Drawing for the job (mm, zero at the part's lowest x, y, z). Coordinates: 2 decimals unless noted, no trailing zeros. Write each loop counter-clockwise with the first axis right and the second up, starting at its lowest first coordinate (ties: lowest second). Pieces come first, ordered by that corner, then holes. Notation, with made-up numbers: (50, 33) - (67, 33) arc R26 cw to (67, 49) - close; hole circle Ø3 at (-34.5, -31.75). An arc over 180 degrees is marked (long way). Write each question's results on one line, items separated by ' | '.
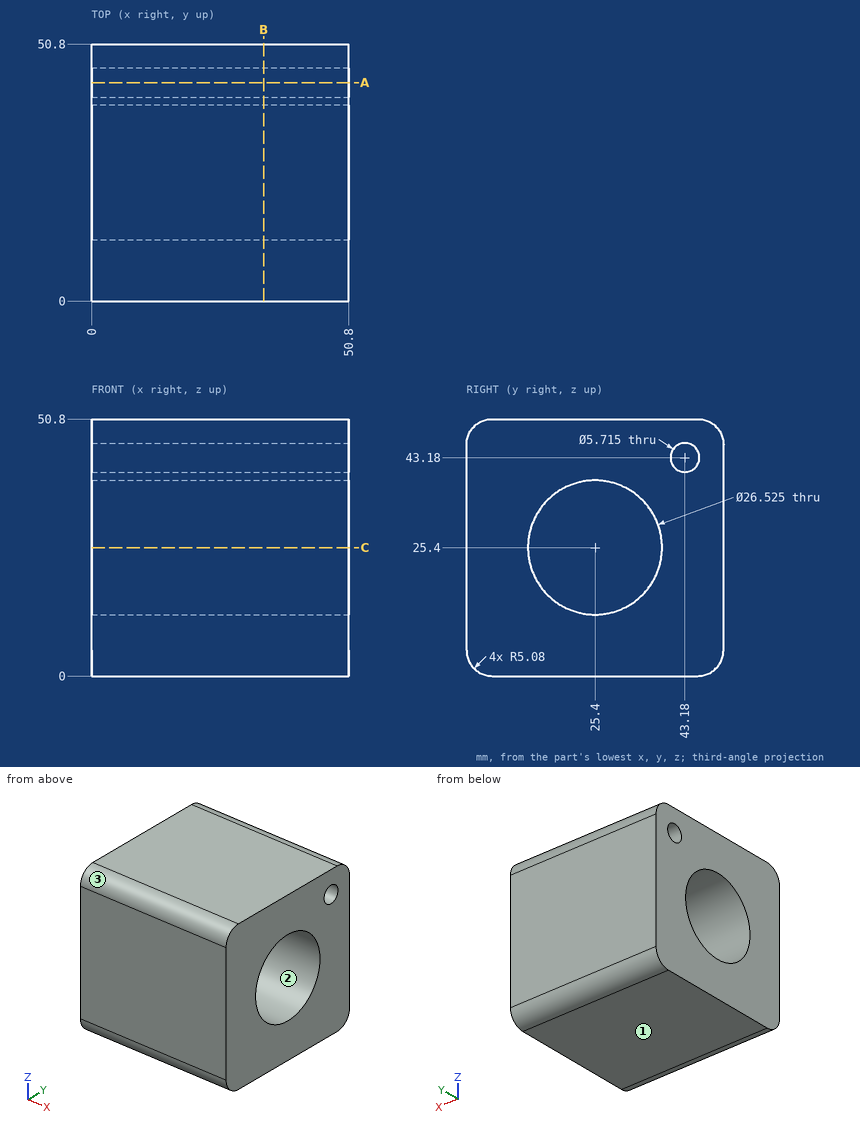
(1) Saw through at A-A on y = 43.18. Write the cut outline in (x, z), then the cut area to 3 significant figures.
Return value:
outline: (0, 0) - (50.8, 0) - (50.8, 40.32) - (0, 40.32) - close; (0, 46.04) - (50.8, 46.04) - (50.8, 50.8) - (0, 50.8) - close | area: 2,290 mm^2
(2) Saw through at B-B on x = 34. Write the cut outline in (y, z) (1 decimal), then the cut area to 3 significant figures.
Return value:
outline: (0, 5.1) arc R5.1 ccw to (5.1, 0) - (45.7, 0) arc R5.1 ccw to (50.8, 5.1) - (50.8, 45.7) arc R5.1 ccw to (45.7, 50.8) - (5.1, 50.8) arc R5.1 ccw to (0, 45.7) - close; hole circle Ø26.5 at (25.4, 25.4); hole circle Ø5.7 at (43.2, 43.2) | area: 1,980 mm^2
(3) Wall check: line 1 (Z direction, x = 20, y = 43); line 2 (Y direction, x = 5.5, z = 43.5); line 3 (Z direction, x = 16, y = 25). Give the ranges that are in metal, low to high. Write a range as from..to.
Return value:
line 1: z = 0..40.33, 46.03..50.8 | line 2: y = 0..40.34, 46.02..50.8 | line 3: z = 0..12.14, 38.66..50.8
(4) Two-plate mould, pull along Y, no slides. Class the marked faces 1, 2 and 3: released by +Y, released by -Y, zero draft, split by the parting line, or undercut.
Return value:
face 1: zero draft | face 2: undercut | face 3: released by -Y
(5) Flat gauge pin, fed straight in: P1, Ø24, axis at y = 25.4, z = 25.4, coming from the +X side. Where does the tip first touch, or does it go through?
Return value:
P1: passes through
(6) Saw through at C-C on z = 25.4. Write the cut outline in (x, y).
Return value:
outline: (0, 0) - (50.8, 0) - (50.8, 12.14) - (0, 12.14) - close; (0, 38.66) - (50.8, 38.66) - (50.8, 50.8) - (0, 50.8) - close
